Design review of the part built by this model. Coordinates are the model's own, in mm. Coordinates: 2 decimals unless noted, no trailing zeros. Write each loop counter-clockwise with the first axis right and the second up, starting at its lowest first coordinate (ties: lowest second). Pieces come first, ordered by that corner, then holes. Notation, with made-up numbers: (-5.5, -30.5) -> (13.5, -30.5) arc R17 cw to (13.5, -9.5) -> close; hole circle Ø8 at (74, 43). An arc over 180 degrees is marked (long way). One line per question, with ' | ' between items. Start each with the question number.
Q1. Add section B-B on z = 1.3. Give the number of separate pieces and of enclosed holes in the cut face, and give its area (3 significant figures).
Q2. Add section D-D on x = -78. State the section outline as (y, z) points, and give its area (3 significant figures).
Q3. Add section A-A on y = -63. State the section outline as (x, z) points, and give its area (3 significant figures).
Q4. Add section C-C on y = 64. State the section outline as (x, z) points.
Q5. Wall thickness on probe 1 along Y at (x, z) = (33.5, 2.4); probe 2 along X at (y, z) = (-30, 1.65); probe 3 along X at (y, z) = (-60, 2.3): over which ranges is each line inside the solid? List them lowest first.
Q6. For P1, Ø0.9, axis at x = 76.5, z = 1, coming from the -Y side; P2, Ø0.9, axis at x = -25, z = 1, coming from the +Y side; P3, Ø1.5, axis at x = -35, z = 2, coming from the +Y side, all flat-tipped, find the tip position at first contact; note any pin that passes through.
from build123d import *

# Parameters (mm, degrees)
IZIM1_W                     = 13.5
IZIM1_H                     = 2.5
Y_KSEKLIK_EKSTR_ZYON1_DEPTH = 3


with BuildPart() as part:
    # Çizim1 → Yükseklik-Ekstrüzyon1 (new body)
    with BuildSketch(Plane.XY):
        with BuildLine():
            Line((-17.5, 72), (-17.5, 55.5))
            ThreePointArc((-17.5, 55.5), (-18.378679656, 53.378679656), (-20.5, 52.5))
            Line((-20.5, 52.5), (-31.5, 52.5))
            Line((-31.5, 52.5), (-31.5, 51))
            Line((-31.5, 51), (-45, 51))
            Line((-45, 51), (-45, 52.5))
            Line((-45, 52.5), (-91.5, 52.5))
            ThreePointArc((-91.5, 52.5), (-93.621320344, 53.378679656), (-94.5, 55.5))
            Line((-94.5, 55.5), (-94.5, 75))
            Line((-94.5, 75), (-95.327166962, 75))
            ThreePointArc((-95.327166962, 75), (-97.34366518, 74.575339872), (-99.01763284, 73.373493976))
            ThreePointArc((-99.01763284, 73.373493976), (-127.5, 0), (-99.01763284, -73.373493976))
            ThreePointArc((-99.01763284, -73.373493976), (-97.34366518, -74.575339872), (-95.327166962, -75))
            Line((-95.327166962, -75), (-94.5, -75))
            Line((-94.5, -75), (-94.5, -55.5))
            ThreePointArc((-94.5, -55.5), (-93.621320344, -53.378679656), (-91.5, -52.5))
            Line((-91.5, -52.5), (-45, -52.5))
            Line((-45, -52.5), (-45, -51))
            Line((-45, -51), (-31.5, -51))
            Line((-31.5, -51), (-31.5, -52.5))
            Line((-31.5, -52.5), (-20.5, -52.5))
            ThreePointArc((-20.5, -52.5), (-18.378679656, -53.378679656), (-17.5, -55.5))
            Line((-17.5, -55.5), (-17.5, -72))
            ThreePointArc((-17.5, -72), (-16.621320344, -74.121320344), (-14.5, -75))
            Line((-14.5, -75), (14.5, -75))
            ThreePointArc((14.5, -75), (16.621320344, -74.121320344), (17.5, -72))
            Line((17.5, -72), (17.5, -55.5))
            ThreePointArc((17.5, -55.5), (18.378679656, -53.378679656), (20.5, -52.5))
            Line((20.5, -52.5), (31.5, -52.5))
            Line((31.5, -52.5), (31.5, -51))
            Line((31.5, -51), (45, -51))
            Line((45, -51), (45, -52.5))
            Line((45, -52.5), (91.5, -52.5))
            ThreePointArc((91.5, -52.5), (93.621320344, -53.378679656), (94.5, -55.5))
            Line((94.5, -55.5), (94.5, -75))
            Line((94.5, -75), (95.327166962, -75))
            ThreePointArc((95.327166962, -75), (97.34366518, -74.575339872), (99.01763284, -73.373493976))
            ThreePointArc((99.01763284, -73.373493976), (127.5, 0), (99.01763284, 73.373493976))
            ThreePointArc((99.01763284, 73.373493976), (97.34366518, 74.575339872), (95.327166962, 75))
            Line((95.327166962, 75), (94.5, 75))
            Line((94.5, 75), (94.5, 55.5))
            ThreePointArc((94.5, 55.5), (93.621320344, 53.378679656), (91.5, 52.5))
            Line((91.5, 52.5), (45, 52.5))
            Line((45, 52.5), (45, 51))
            Line((45, 51), (31.5, 51))
            Line((31.5, 51), (31.5, 52.5))
            Line((31.5, 52.5), (20.5, 52.5))
            ThreePointArc((20.5, 52.5), (18.378679656, 53.378679656), (17.5, 55.5))
            Line((17.5, 55.5), (17.5, 72))
            ThreePointArc((17.5, 72), (16.621320344, 74.121320344), (14.5, 75))
            Line((14.5, 75), (-14.5, 75))
            ThreePointArc((-14.5, 75), (-16.621320344, 74.121320344), (-17.5, 72))
        make_face()
        with Locations((38.25, 30.75)):
            Rectangle(IZIM1_W, IZIM1_H, mode=Mode.SUBTRACT)
        with Locations((-38.25, -30.75)):
            Rectangle(IZIM1_W, IZIM1_H, mode=Mode.SUBTRACT)
        with Locations((-38.25, 30.75)):
            Rectangle(IZIM1_W, IZIM1_H, mode=Mode.SUBTRACT)
        with Locations((38.25, -30.75)):
            Rectangle(IZIM1_W, IZIM1_H, mode=Mode.SUBTRACT)
    extrude(amount=Y_KSEKLIK_EKSTR_ZYON1_DEPTH)


solid = part.part
Output values:
1) separate pieces: 1 | enclosed holes: 4 | area: 28,300 mm2
2) outline: (-52.5, 0) -> (52.5, 0) -> (52.5, 3) -> (-52.5, 3) -> close | area: 315 mm2
3) outline: (-107.39, 0) -> (-94.5, 0) -> (-94.5, 3) -> (-107.39, 3) -> close; (-17.5, 0) -> (17.5, 0) -> (17.5, 3) -> (-17.5, 3) -> close; (94.5, 0) -> (107.39, 0) -> (107.39, 3) -> (94.5, 3) -> close | area: 182 mm2
4) outline: (-106.67, 0) -> (-94.5, 0) -> (-94.5, 3) -> (-106.67, 3) -> close; (-17.5, 0) -> (17.5, 0) -> (17.5, 3) -> (-17.5, 3) -> close; (94.5, 0) -> (106.67, 0) -> (106.67, 3) -> (94.5, 3) -> close
5) probe 1: y = -51 to -32, -29.5 to 29.5, 32 to 51 | probe 2: x = -123.28 to -45, -31.5 to 31.5, 45 to 123.28 | probe 3: x = -109.45 to -94.5, -17.5 to 17.5, 94.5 to 109.45
6) P1: stops at y = -52.5 | P2: stops at y = 52.5 | P3: stops at y = 51
